Model file for the job. Use its own axes, mm. Face numbers are marked on the shaded views. Give positions to 0.01 mm unless a question says otherwise; leave off trailing zeros. Write each loop counter-clockwise with the first axis right and the second up, starting at its lowest first coordinate (ties: lowest second). Pieces come first, ordered by that corner, then holes.
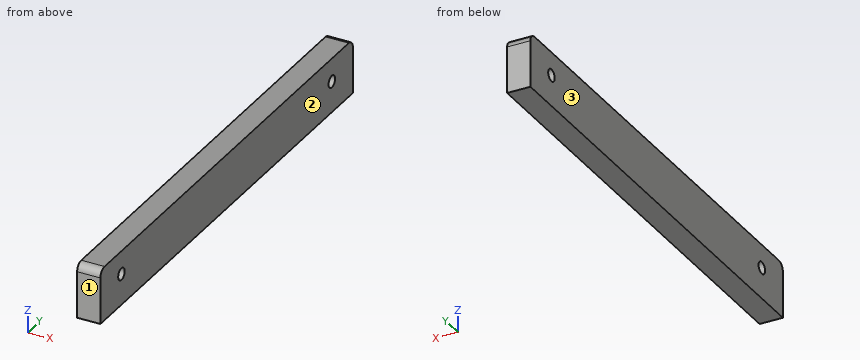
```python
from build123d import *

# Parameters (mm, degrees)
SKETCH1_W           = 14
SKETCH1_H           = 120
SKETCH1_R           = 1.55
BOSS_EXTRUDE1_DEPTH = 6
FILLET1_R           = 2


with BuildPart() as part:
    # Sketch1 → Boss-Extrude1 (new body)
    with BuildSketch(Plane(origin=(0, 0, 0), x_dir=(0, 0, -1), z_dir=(1, 0, 0))):
        with Locations((-7, 0)):
            Rectangle(SKETCH1_W, SKETCH1_H)
        with Locations((-8, 50)):
            Circle(SKETCH1_R, mode=Mode.SUBTRACT)
        with Locations(Location((-8, -50, 0), (0, 0, 180))):
            Circle(SKETCH1_R, mode=Mode.SUBTRACT)
    extrude(amount=BOSS_EXTRUDE1_DEPTH)

    # Fillet1
    fillet1_edges = [part.edges().sort_by_distance(p)[0] for p in [
        (3, -60, 14),
        (3, 60, 14),
    ]]
    fillet(fillet1_edges, radius=FILLET1_R)


solid = part.part
```
1. Slice it at A-A, the plane z = 8. Write the cut outline in (x, y).
Calculated:
outline: (0, -60) - (6, -60) - (6, -51.55) - (0, -51.55) - close; (0, -48.45) - (6, -48.45) - (6, 48.45) - (0, 48.45) - close; (0, 51.55) - (6, 51.55) - (6, 60) - (0, 60) - close
2. Pin check, flat tip, straight feed: P1, Ø3, axis at y = -50, z = 8, coming from the +X side. Stop position of the tip, or through.
Calculated:
P1: passes through
3. Pull direction X, two halves, no side cores. Call the marked faces 1, 2 and 3: +X half, -X half, draft (parallel to the pull), parting line (faces both ways), or undercut.
Calculated:
face 1: draft
face 2: +X half
face 3: -X half
4. Probe probe 1 along Y at (x, z) = (3, 8); probe 2 along Z at (x, y) = (2.95, -50); probe 3 along Z at (x, y) = (4.8, 51). List the from-to ranges inside material, lowest first.
Calculated:
probe 1: y = -60 to -51.55, -48.45 to 48.45, 51.55 to 60
probe 2: z = 0 to 6.45, 9.55 to 14
probe 3: z = 0 to 6.82, 9.18 to 14
5. Slice it at B-B, the plane y = -50. Write the cut outline in (x, z), and give its area (3 significant figures).
Calculated:
outline: (0, 0) - (6, 0) - (6, 6.45) - (0, 6.45) - close; (0, 9.55) - (6, 9.55) - (6, 14) - (0, 14) - close
area: 65.4 mm2
